Source: CAD feature listing. Evaluate the final solid. Frame: model axes, mm. A direction names the side the tool comes from. Round coordinates to 2 decimals unless told otherwise and drop trailing zeros. Loops run counter-clockwise (first coordinate to the right, second up) from the corner with the lowest first, then second, coordinate; pieces in that order, holes last.
(1) Section A-A, the plane x = 41. Return the cut outline in (y, z).
(2) First-contact query: pin 1 Ø1.5 at (x, z) = (49.5, 1.5) entering from +Y. Flat tip, straight axial feed; report the tip coordinate or a pass-through.
(3) Material intervals for probe 1 along X at (y, z) = (-3.25, 5); probe 2 along Y at (x, z) = (63.5, -3); probe 3 along Z at (x, y) = (31.5, -1), sorted ascending.
(4) Set-up query: faces 1 (the flat face through (0, 5, 2)), 2 (the conical face through (-6.226, 4.133, -7.199)). Return all of +Z, -Z, +X, -X, +Y, -Y with unobstructed straight access to the full face (end or side cutting, diameter ignored); none if empty.
Autodesk Inventor part; units mm, degrees
ref_plane "Work Plane1" through (1.525, 0, 0) normal (0, 0, 1) x (1, 0, 0)
ref_plane "YZ Plane" through (0, 0, 0) normal (1, 0, 0) x (0, 1, 0)
ref_plane "XZ Plane" through (0, 0, 0) normal (0, 1, 0) x (-1, 0, 0)
sketch "Sketch1" plane through (0, 0, 0) normal (0, 0, 1) x (1, 0, 0)
  line L0 (0, 7.315) -> (0, 5)
  line L1 (54, 5) -> (80, 5)
  line L2 (80, 5) -> (80, 0)
  line L3 (80, 0) -> (-0.6001, 0)
  line L4 (-16.7201, 0) -> (96.12, 0)
  line L5 (-0.6001, 0) -> (-0.6001, 7.315)
  line L6 (-0.6001, 7.315) -> (0, 7.315)
  line L7 (54, 5) -> (53.0797, 5)
  line L8 (53.0797, 5) -> (0, 5)
  line L9 (0, -1.463) -> (0, 8.778)
  dimension "d0" = 80
  dimension "d1" = 26
  dimension "d2" = 10
  dimension "d9" = 0.6001
  dimension "d10" = 14.63
  dimension "d13" = 0.9203
  dimension "d14" = 10
revolve "Body" add sketch "Sketch1" angle 360 about axis through (80, 0, 0) along (-1, 0, 0)
sketch "Sketch2" plane through (-0.6001, 0, 0) normal (-1, 0, 0) x (0, 0, 1)
  line L0 (0, 9.2376) -> (8, 4.6188)
  line L1 (8, 4.6188) -> (8, -4.6188)
  line L2 (8, -4.6188) -> (0, -9.2376)
  line L3 (0, -9.2376) -> (-8, -4.6188)
  line L4 (-8, -4.6188) -> (-8, 4.6188)
  line L5 (-8, 4.6188) -> (0, 9.2376)
  point P0 (0, 0)
  point P1 (0, 0)
  dimension "d11" = 16
extrude "Head" add sketch "Sketch2" along normal blind 5.8
sketch "Sketch4" plane through (0, 0, 0) normal (0, 0, 1) x (1, 0, 0)
  line L0 (-6.4001, 8) -> (-6.4001, 9.2376)
  line L1 (-6.4001, 9.2376) -> (-5.6856, 9.2376)
  line L2 (-5.6856, 9.2376) -> (-6.4001, 8)
  line L3 (-7.5601, 0) -> (0.5599, 0)
  line L4 (-0.6001, 9.2376) -> (-6.4001, 9.2376)
  line L5 (-6.4001, 4.6188) -> (-6.4001, 9.2376)
  dimension "d5" = 30
  dimension "d19" = 16
revolve "Chamfer1" cut sketch "Sketch4" angle 360 about axis through (-10, 0, 0) along (1, 0, 0)
thread "Thread"
chamfer "Chamfer2" distance 0.9202 distance2 0.9203 1 edges at (80, -5, 0) measured on face at (80, 0.2493, 1.2557)
ref_plane "Work Plane1" through (1.525, 0, 0) normal (0, 0, 1) x (1, 0, 0)
equation "\"d0\" = NLG"
equation "\"d1\" = GEL"
equation "\"d2\" = GD"
equation "\"d10\" = SD2"
equation "\"d14\" = BDM"
equation "\"d11\" = SW"
equation "\"d3\" = KOH - SD"
equation "\"d5\" = ANG1"
equation "\"d19\" = SW0"
equation "\"d15\" = GEL"
equation "\"d6\" = -0.5 * SPD + 0.5 * GD"
equation "\"NLG\" = 80"
equation "\"GD\" = NND"
equation "\"BDM\" = NND"
equation "\"KOH\" = 6.4"
equation "\"GEL\" = 26"
equation "\"SW\" = 16"
equation "\"SW0\" = SW"
equation "\"SPD\" = NND - 1.2269 * PTC"
equation "\"SD2\" = 14.63"
equation "\"SD\" = 0.6"
equation "\"ANG1\" = 30deg"
equation "\"GAL\" = 0.61345 * PTC"
equation "\"GUL\" = 0.61345 * PTC"
equation "\"RR\" = 0.4"
equation "\"GD1\" = THREADDIA - 1.2269 * PTC"
equation "\"SDH\" = SD2"
equation "\"TOA\" = 30deg"
equation "\"PTC\" = 1.5"
equation "\"E0\" = 1.155 * SW"
properties part number "ISO 4014 - M10 x 80" material "Stainless Steel, 440C"
Output values:
1. outline: circle Ø10 at (0, 0)
2. pin 1: stops at y = 4.94
3. probe 1: x = -6.4 to 0
3. probe 2: y = -4 to 4
3. probe 3: z = -4.9 to 4.9
4. face 1: +X
4. face 2: -Z, -X, +Y
